Can you work these out from the model? Positions are in its coordinate system, mm. Face numbers are marked on the shaded views. A direction names the side the tool comes from. Coordinates: 2 decimals unless noted, no trailing zeros. Order: outer loops, then holes, each group sorted by start corner. A loop starts at its lowest first (then second) coordinate and runs counter-clockwise, first axis right, second up. Notation, with made-up numbers: M 21,6.25 L 49,6.25 A21 cw 49,36.25 Z; hole C -28.75,-20 d1. An arc over 180 degrees is marked long. Answer as a JSON object with one key per item and string values.
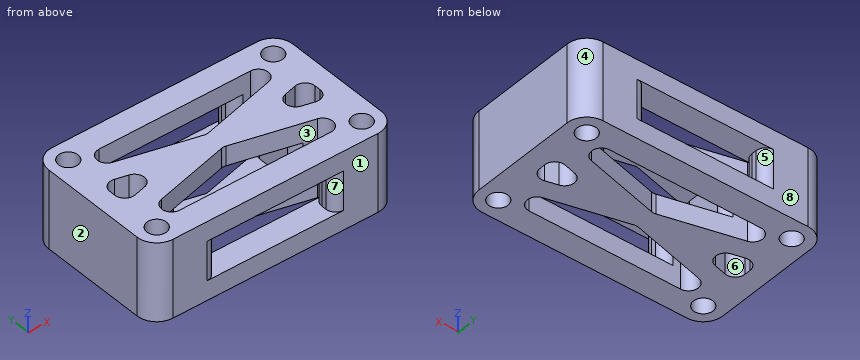
from build123d import *

# Parameters (mm, degrees)
SKETCH_1_W               = 25
SKETCH_1_H               = 15
EXTRUDE_1_DEPTH          = 8
FILLET_4_R               = 2
CUT_EXTRUDE_3_DEPTH      = 10
SKETCH_3_R               = 1
CUT_EXTRUDE_4_DEPTH      = 10
CUT_EXTRUDE_5_DEPTH      = 22.100947846
CUT_EXTRUDE_5_DEPTH_BACK = 22.100947846
SKETCH_4_W               = 12
SKETCH_4_H               = 4
FILLET_6_R               = 1


with BuildPart() as part:
    # 草图1 → 凸台-拉伸1 (new body)
    with BuildSketch(Plane.XY):
        Rectangle(SKETCH_1_W, SKETCH_1_H)
    extrude(amount=EXTRUDE_1_DEPTH)

    # 圆角4
    fillet_4_edges = [part.edges().sort_by_distance(p)[0] for p in [
        (12.5, -7.5, 4),
        (-12.5, -7.5, 4),
        (-12.5, 7.5, 4),
        (12.5, 7.5, 4),
    ]]
    fillet(fillet_4_edges, radius=FILLET_4_R)

    # 草图2 → 切除-拉伸3 (cut)
    with BuildSketch(Plane.XY.offset(8)):
        with BuildLine():
            Line((-0.242535625, -1.091410313), (-7.996324374, -3.0298575))
            ThreePointArc((-7.996324374, -3.0298575), (-8.746296305, -4.122183264), (-7.753788749, -5))
            Line((-7.753788749, -5), (7.753788749, -5))
            ThreePointArc((7.753788749, -5), (8.746296305, -4.122183264), (7.996324374, -3.0298575))
            Line((7.996324374, -3.0298575), (0.242535625, -1.091410313))
            ThreePointArc((0.242535625, -1.091410313), (0, -1.061552813), (-0.242535625, -1.091410313))
        make_face()
        with BuildLine():
            Line((7.753788749, 5), (-7.753788749, 5))
            ThreePointArc((-7.753788749, 5), (-8.746296305, 4.122183264), (-7.996324374, 3.0298575))
            Line((-7.996324374, 3.0298575), (-0.242535625, 1.091410313))
            ThreePointArc((-0.242535625, 1.091410313), (0, 1.061552813), (0.242535625, 1.091410313))
            Line((0.242535625, 1.091410313), (7.996324374, 3.0298575))
            ThreePointArc((7.996324374, 3.0298575), (8.746296305, 4.122183264), (7.753788749, 5))
        make_face()
        with BuildLine():
            Line((-9.257464375, -1.283589687), (-8.003675626, -0.9701425))
            ThreePointArc((-8.003675626, -0.9701425), (-7.246211251, 0), (-8.003675626, 0.9701425))
            Line((-8.003675626, 0.9701425), (-9.257464375, 1.283589687))
            ThreePointArc((-9.257464375, 1.283589687), (-10.115412209, 1.101652625), (-10.5, 0.313447187))
            Line((-10.5, 0.313447187), (-10.5, -0.313447187))
            ThreePointArc((-10.5, -0.313447187), (-10.115412209, -1.101652625), (-9.257464375, -1.283589687))
        make_face()
        with BuildLine():
            Line((10.5, 0.313447187), (10.5, -0.313447187))
            ThreePointArc((10.5, -0.313447187), (10.115412209, -1.101652625), (9.257464375, -1.283589687))
            Line((9.257464375, -1.283589687), (8.003675626, -0.9701425))
            ThreePointArc((8.003675626, -0.9701425), (7.246211251, 0), (8.003675626, 0.9701425))
            Line((8.003675626, 0.9701425), (9.257464375, 1.283589687))
            ThreePointArc((9.257464375, 1.283589687), (10.115412209, 1.101652625), (10.5, 0.313447187))
        make_face()
    extrude(amount=-CUT_EXTRUDE_3_DEPTH, mode=Mode.SUBTRACT)

    # 草图3 → 切除-拉伸4 (cut)
    with BuildSketch(Plane.XY.offset(8)):
        with Locations((-10.5, 5.5)):
            Circle(SKETCH_3_R)
        with Locations(Location((10.5, 5.5, 0), (0, 0, 180))):
            Circle(SKETCH_3_R)
        with Locations((10.5, -5.5)):
            Circle(SKETCH_3_R)
        with Locations(Location((-10.5, -5.5, 0), (0, 0, 180))):
            Circle(SKETCH_3_R)
    extrude(amount=-CUT_EXTRUDE_4_DEPTH, mode=Mode.SUBTRACT)

    # 草图4 → 切除-拉伸5 (cut, two sides: drawn at the far end of the back side and taken through both)
    with BuildSketch(Plane.XZ.offset(7.5).offset(-CUT_EXTRUDE_5_DEPTH_BACK)):
        with Locations((0, 4)):
            Rectangle(SKETCH_4_W, SKETCH_4_H)
    extrude(amount=CUT_EXTRUDE_5_DEPTH + CUT_EXTRUDE_5_DEPTH_BACK, mode=Mode.SUBTRACT)

    # 圆角6
    fillet_6_edges = [part.edges().sort_by_distance(p)[0] for p in [
        (6, 2.530776406, 4),
        (-6, 5, 4),
        (-6, -7.5, 4),
        (-6, -5, 4),
        (-6, -2.530776406, 4),
        (-6, 2.530776406, 4),
        (-6, 7.5, 4),
        (6, -7.5, 4),
        (6, -5, 4),
        (6, -2.530776406, 4),
        (6, 5, 4),
        (6, 7.5, 4),
    ]]
    fillet(fillet_6_edges, radius=FILLET_6_R)


solid = part.part
Item 1: I want a section at C-C, the plane x = 2. Write out the boundary of the cut face in (y, z).
Answers follow:
{"outline": "M -7.5,0 L -5,0 L -5,2 L -7.5,2 Z; M -7.5,6 L -5,6 L -5,8 L -7.5,8 Z; M -1.53,0 L 1.53,0 L 1.53,2 L -1.53,2 Z; M -1.53,6 L 1.53,6 L 1.53,8 L -1.53,8 Z; M 5,0 L 7.5,0 L 7.5,2 L 5,2 Z; M 5,6 L 7.5,6 L 7.5,8 L 5,8 Z"}
Item 2: I want a section at A-A, the plane y = 0. Write out the boundary of the cut face in (x, z).
Answers follow:
{"outline": "M -12.5,0 L -10.5,0 L -10.5,8 L -12.5,8 Z; M -7.25,0 L 7.25,0 L 7.25,8 L -7.25,8 Z; M 10.5,0 L 12.5,0 L 12.5,8 L 10.5,8 Z; hole M -6,2 L 6,2 L 6,6 L -6,6 Z"}
Item 3: I want a section at B-B, the plane z = 2.5. Give the number of separate pieces and of enclosed holes in the cut face, plus the area to 3 significant figures.
Answers follow:
{"separate pieces": "2", "enclosed holes": "6", "area": "141 mm^2"}
Item 4: If we mould it in two halves opening along X, with no side actions, what happens to the marked faces 1, 2, 3 and 4? For each: pulls with the +X half, pulls with the -X half, needs draft (parallel to the pull), parting line crosses it, or undercut.
Answers follow:
{"face 1": "needs draft", "face 2": "pulls with the -X half", "face 3": "undercut", "face 4": "pulls with the +X half"}
Item 5: Which directions (+Z, -Z, +X, -X, +Y, -Y) give clear straight access to the entire face, cutting with the end or side of a thin tool? Please do the marked faces 5, 6, 7 and 8.
Answers follow:
{"face 5": "+Y", "face 6": "+Z, -Z", "face 7": "-Y", "face 8": "+Z, -Z, +X, -X, +Y"}
Item 6: Please list where these lines run through material, in increasing order: line 1 (Z direction, x = -3.5, y = 0); line 2 (Y direction, x = -8, z = 2.5); line 3 (X direction, y = -1.75, z = 3.5).
Answers follow:
{"line 1": "z = 0 to 2, 6 to 8", "line 2": "y = -7.5 to -4.97, -3.03 to -0.97, 0.97 to 3.03, 4.97 to 7.5", "line 3": "x = -12.5 to -6, 6 to 12.5"}
Item 7: I want a section at D-D, the plane y = 4.25. Write out the boundary of the cut face in (x, z), plus the area to 3 significant figures.
Answers follow:
{"outline": "M -12.5,0 L -8.72,0 L -8.72,8 L -12.5,8 Z; M 8.72,0 L 12.5,0 L 12.5,8 L 8.72,8 Z", "area": "60.4 mm^2"}
